Check sheet for the drawn part. Datum: minimum x, y, z corner. Units: mm. A direction names the side the tool comes from. Coordinates: 2 decimals unless noted, no trailing zeros. Order: outer loops, then holes, each group sorted by start corner. A loop starts at its lowest first (then second) coordinate and runs counter-clockwise, first axis right, second up.
1. Thickness scan on line 1 (Y direction, x = 31.7, z = 8.7); line 2 (Y direction, x = 20, z = 8.2); line 3 (X direction, y = 58, z = 5.75). Record the ranges inside material, lowest first.
2. Cross-section at C-C (z = 2.5). Enter the section's corners in (x, y), then the cut area to 3 significant figures.
3. Draft check along Y on the marked faces 4, 5 and 6. Enter one of: released by +Y, released by -Y, zero draft, split by the parting line, or undercut.
4. Set-up check for the marked faces 1, 2 and 3: record each of +Z, -Z, +X, -X, +Y, -Y from which the full face is reachable in a straight line by a thin tool's end or side.
5. Cross-section at D-D (y = 38.3). Enter the section's corners in (x, z).
6. Gauge pin test, flat end, axial feed: pin 1 Ø8 at (x, y) = (20, 15) entering from -Z. Record the tip position at first contact, or that the pin passes through.
7. Cross-section at B-B (x = 31.7). Enter the section's corners in (y, z).
8. Cross-section at A-A (y = 85). Enter the section's corners in (x, z), then the cut area to 3 significant figures.
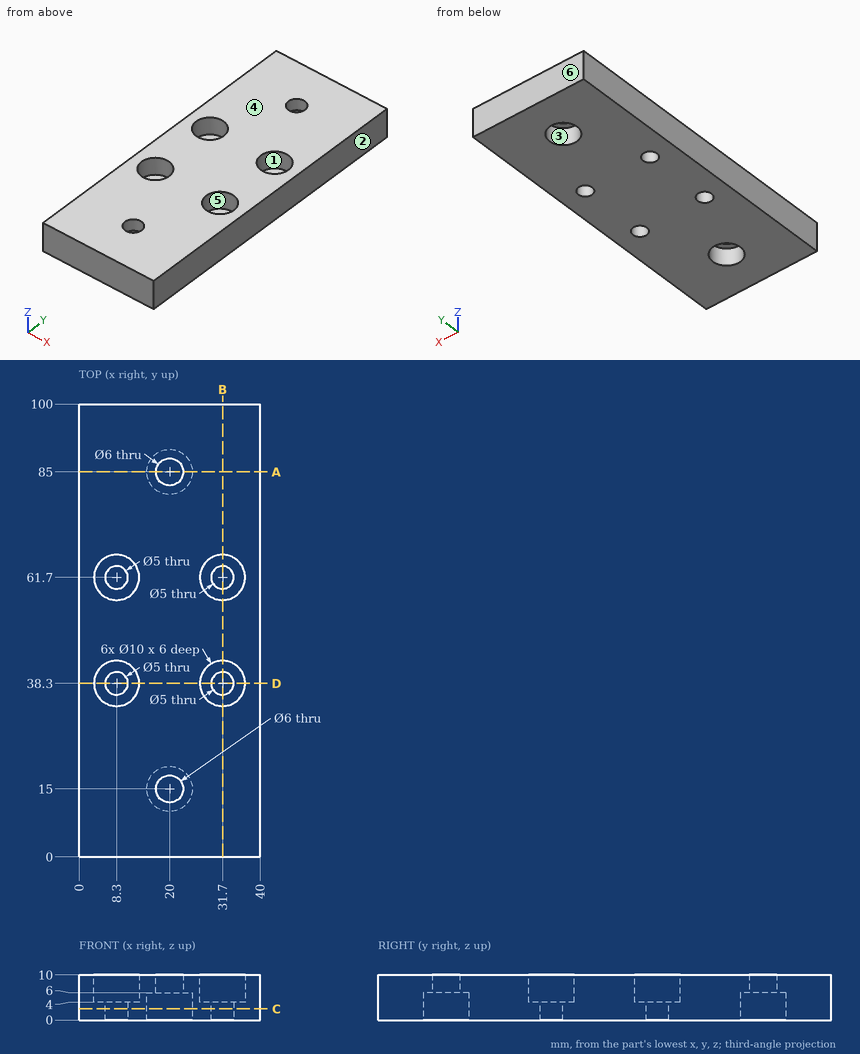
Data:
1. line 1: y = 0 to 33.3, 43.3 to 56.7, 66.7 to 100
1. line 2: y = 0 to 12, 18 to 82, 88 to 100
1. line 3: x = 0 to 4.94, 11.66 to 28.34, 35.06 to 40
2. outline: (0, 0) - (40, 0) - (40, 100) - (0, 100) - close; hole circle Ø5 at (8.3, 38.3); hole circle Ø5 at (8.3, 61.7); hole circle Ø10 at (20, 15); hole circle Ø10 at (20, 85); hole circle Ø5 at (31.7, 38.3); hole circle Ø5 at (31.7, 61.7)
2. area: 3,760 mm2
3. face 4: zero draft
3. face 5: undercut
3. face 6: released by +Y
4. face 1: +Z
4. face 2: +Z, -Z, +X, +Y, -Y
4. face 3: -Z
5. outline: (0, 0) - (5.8, 0) - (5.8, 4) - (3.3, 4) - (3.3, 10) - (0, 10) - close; (10.8, 0) - (29.2, 0) - (29.2, 4) - (26.7, 4) - (26.7, 10) - (13.3, 10) - (13.3, 4) - (10.8, 4) - close; (34.2, 0) - (40, 0) - (40, 10) - (36.7, 10) - (36.7, 4) - (34.2, 4) - close
6. pin 1: stops at z = 6
7. outline: (0, 0) - (35.8, 0) - (35.8, 4) - (33.3, 4) - (33.3, 10) - (0, 10) - close; (40.8, 0) - (59.2, 0) - (59.2, 4) - (56.7, 4) - (56.7, 10) - (43.3, 10) - (43.3, 4) - (40.8, 4) - close; (64.2, 0) - (100, 0) - (100, 10) - (66.7, 10) - (66.7, 4) - (64.2, 4) - close
8. outline: (0, 0) - (15, 0) - (15, 6) - (17, 6) - (17, 10) - (0, 10) - close; (23, 6) - (25, 6) - (25, 0) - (40, 0) - (40, 10) - (23, 10) - close
8. area: 316 mm2
